Autodesk Inventor part; units mm, degrees
ref_plane "YZ Plane" through (0, 0, 0) normal (1, 0, 0) x (0, 1, 0)
ref_plane "XZ Plane" through (0, 0, 0) normal (0, 1, 0) x (-1, 0, 0)
ref_plane "XY Plane" through (0, 0, 0) normal (0, 0, 1) x (1, 0, 0)
sketch "스케치1" plane through (0, 0, 0) normal (0, 0, 1) x (1, 0, 0)
  line L0 (-22.85, 14) -> (53.375, 14)
  arc A0 (-22.85, 14) -> (-34.1366, 8.2833) centre (-22.85, 0) ccw
  arc A1 (-34.1366, 8.2833) -> (-32.5242, 5.1) centre (-32.5242, 7.1) ccw
  line L1 (-22.85, 5.1) -> (-32.5242, 5.1)
  arc A2 (-22.85, -5.1) -> (-22.85, 5.1) centre (-22.85, 0) ccw
  line L2 (-32.5242, -5.1) -> (-22.85, -5.1)
  arc A3 (-32.5242, -5.1) -> (-34.1366, -8.2833) centre (-32.5242, -7.1) ccw
  arc A4 (-34.1366, -8.2833) -> (-22.85, -14) centre (-22.85, 0) ccw
  line L3 (53.375, -14) -> (-22.85, -14)
  line L4 (53.375, 14) -> (53.375, -14)
  circle A5 centre (-15.0718, 7.7782) radius 1.025
  circle A6 centre (-15.0718, -7.7782) radius 1.025
  circle A7 centre (-22.85, -11) radius 1.025
  circle A8 centre (-22.85, 11) radius 1.025
  circle A9 centre (-30.6282, -7.7782) radius 1.025
  circle A10 centre (-11.85, 0) radius 1.025
  circle A11 centre (-30.6282, 7.7782) radius 1.025
  circle A12 centre (50.8741, 11) radius 1.35
  circle A13 centre (50.8741, -11) radius 1.35
  line L5 (53.375, 14) -> (47.375, 14)
  line L6 (47.375, 14) -> (47.375, -14)
  line L7 (47.375, -14) -> (53.375, -14)
  line L8 (53.375, -14) -> (53.375, 14)
  point P0 (0, 0)
  dimension "d0" = 6
extrude "돌출1" add sketch "스케치1" along normal blind 6.3 contours L0 L4 L3 L6
sketch "스케치2" plane through (47.375, -14, 0) normal (-1, 0, 0) x (0, 0, 1)
  line L0 (0, 14) -> (0, 11)
  line L1 (0, 28) -> (0, 0)
  line L2 (-6.2, 17.1) -> (-6.2, 28)
  line L3 (-6.2, 28) -> (0, 28)
  line L4 (-0.2, 17.1) -> (-0.2, 28)
  line L5 (0, 11) -> (-6.2, 11)
  line L6 (-6.2, 11) -> (-6.2, 17)
  line L7 (-6.2, 17) -> (0, 17)
  line L8 (0, 17) -> (0, 11)
  line L9 (-0.2, 17.1) -> (-6.2, 17.1)
  point P0 (-6, 11)
  point P1 (0, 17.1)
  dimension "d3" = 3
extrude "돌출2" add sketch "스케치2" against normal blind 6 contours L0 L5 L6 L7 L1
properties part number "afsd" material "PMMA 플라스틱"
Verification items for the finished model (mm, model axes). A direction names the side the tool comes from. Round coordinates to 2 decimals unless told otherwise and drop trailing zeros. Order: outer loops, then holes, each group sorted by start corner. A loop starts at its lowest first (then second) coordinate and runs counter-clockwise, first axis right, second up.
1. Section check C-C on x = 50.75. Record the cut outline in (y, z).
Final values:
outline: (-14, 0) - (-12.34, 0) - (-12.34, 6.3) - (-14, 6.3) - close; (-9.66, 0) - (-3, 0) - (-3, -6.2) - (3, -6.2) - (3, 0) - (9.66, 0) - (9.66, 6.3) - (-9.66, 6.3) - close; (12.34, 0) - (14, 0) - (14, 6.3) - (12.34, 6.3) - close
2. Go/stop test with flat-tipped pins: P1, Ø3, axis at x = 50, y = 8, coming from the -Z side; P2, Ø3, axis at x = 50, z = -3, coming from the +Y side; P3, Ø1.6, axis at x = 50.87, y = 11, coming from the -Z side. Record where each tip stops, or that it passes through.
Final values:
P1: stops at z = 0
P2: stops at y = 3
P3: passes through
3. Section check A-A on y = 11. Record the cut outline in (x, z) (3 decimals).
Final values:
outline: (47.375, 0) - (49.524, 0) - (49.524, 6.3) - (47.375, 6.3) - close; (52.224, 0) - (53.375, 0) - (53.375, 6.3) - (52.224, 6.3) - close
4. Section check B-B on z = 1. Record the cut outline in (x, y) (3 decimals).
Final values:
outline: (47.375, -14) - (53.375, -14) - (53.375, 14) - (47.375, 14) - close; hole circle Ø2.7 at (50.874, -11); hole circle Ø2.7 at (50.874, 11)
5. Section check D-D on x = 52.75. Record the cut outline in (y, z).
Final values:
outline: (-14, 0) - (-3, 0) - (-3, -6.2) - (3, -6.2) - (3, 0) - (14, 0) - (14, 6.3) - (-14, 6.3) - close
6. Release check for a two-part mould opening along Y. For faces 4 (the flat face through (50, 9, 0)), 5 (the cylindrical face through (49.879, 10.088, 3.106)), 6 (the flat face through (50, 14, 3)) record: +Y half, -Y half, draft (parallel to the pull), parting line (faces both ways), or undercut.
Final values:
face 4: draft
face 5: undercut
face 6: +Y half
7. Access from +Z, -Z, +X, -X, +Y, -Y to the whole of each face (thin tool, end or side, straight path). Record for faces 1 (the flat face through (50, -14, 3)), 2 (the flat face through (50, -3, -3)), 3 (the flat face through (50, 3, -3)).
Final values:
face 1: +Z, -Z, +X, -X, -Y
face 2: -Z, +X, -X, -Y
face 3: -Z, +X, -X, +Y
8. Thickness scan on L1, parallel to Y at x = 51, z = 5; L2, parallel to Y at x = 52.25, z = -0.75; L3, parallel to Z at x = 53, y = 9.25. Record the ranges inside material, lowest first.
Final values:
L1: y = -14 to -12.34, -9.66 to 9.66, 12.34 to 14
L2: y = -3 to 3
L3: z = 0 to 6.3
